Could you check a few things on this drawing? It's one solid part, dimensions in mm from its lowest x, y, z. Give positions to 0.01 mm unless a question says otherwise; leave off trailing zeros. Order: outer loops, then holes, each group sorted by start corner. A loop starts at its lowest first (then second) coordinate and runs counter-clockwise, first axis right, second up. Notation, with made-up numbers: (-19, -8) - (26, -8) arc R4 cw to (26, -4) - close; hole circle Ø8 at (-21.5, 75.25). An arc over 180 degrees is marked (long way). One line per question, with ' | ' between items. Start each with the question number.
1. For P1, Ø5, axis at y = 3.5, z = 7.5, coming from the +X side; P2, Ø2.5, axis at x = 14, z = 13, coming from the +Y side; P3, Ø2, axis at x = 10, y = 9, coming from the -Z side, each with a flat end and sliding along its axis, tell me the tip position at first contact or that it passes through.
2. I need wall thicknesses on probe 1 along X at (y, z) = (14.25, 15); probe 2 along X at (y, z) = (8.25, 15); probe 3 along Z at (x, y) = (17, 15). Which ranges of each line are inside material? Lowest first, please. Write a range as from..to.
3. Imagine slicing it at C-C (x = 7.5). Please give me the cut outline in (y, z).
4. Imagine slicing it at B-B (x = 16.5). Please give me the cut outline in (y, z) (3 decimals), and give its area (3 significant figures).
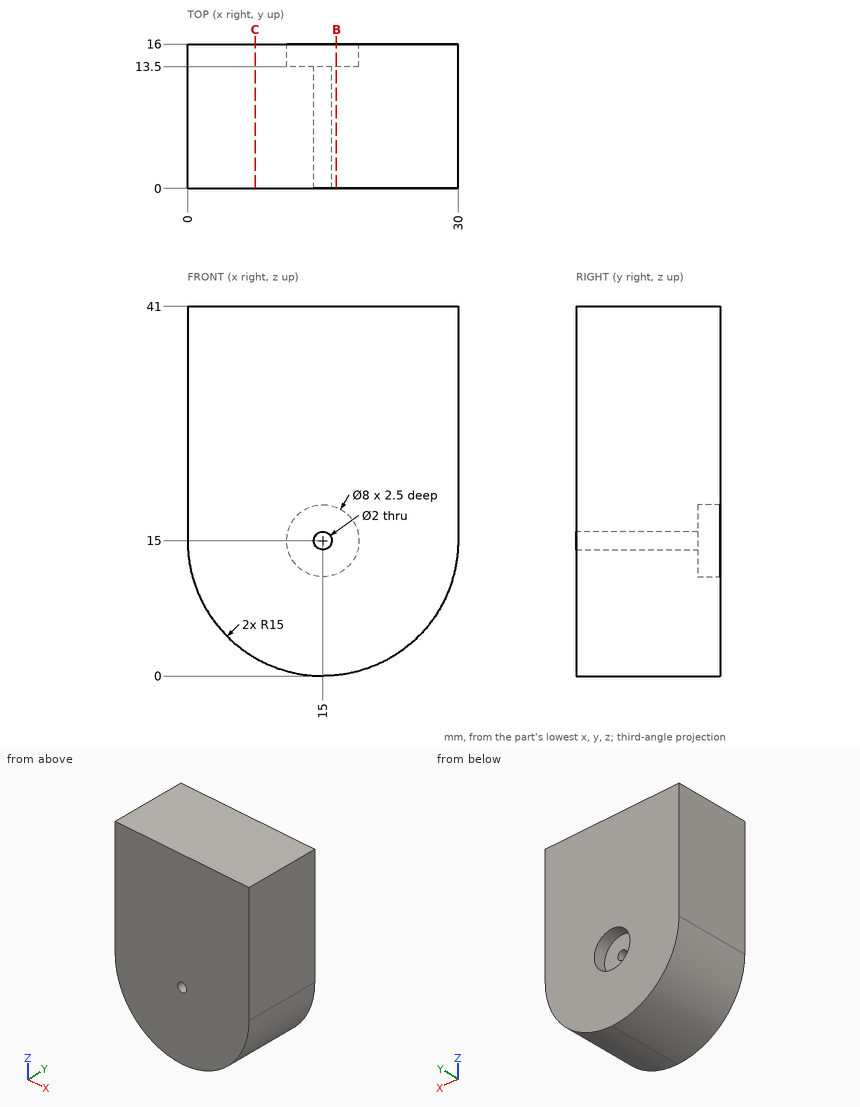
Results found:
1) P1: stops at x = 29.14 | P2: stops at y = 13.5 | P3: stops at z = 0.54
2) probe 1: x = 0..11, 19..30 | probe 2: x = 0..14, 16..30 | probe 3: z = 0.13..11.54, 18.46..41
3) outline: (0, 2.01) - (16, 2.01) - (16, 41) - (0, 41) - close
4) outline: (0, 0.075) - (16, 0.075) - (16, 11.292) - (13.5, 11.292) - (13.5, 18.708) - (16, 18.708) - (16, 41) - (0, 41) - close | area: 636 mm2
